from build123d import *

# Parameters (mm, degrees)
F0_W     = 28
F0_H     = 16
F1_DEPTH = 85
F2_W     = 23
F2_H     = 9
F2_H_2   = 7
F3_DEPTH = 25


with BuildPart() as f1:
    # F0 (on Front) → F1 (new body)
    with BuildSketch(Plane.XZ):
        Rectangle(F0_W, F0_H)
    extrude(amount=F1_DEPTH)

    # F2 (on face) → F3 (cut)
    with BuildSketch(Plane(origin=(0, 0, -8), x_dir=(1, 0, 0), z_dir=(0, 0, -1))):
        with Locations((0, 77.5)):
            Rectangle(F2_W, F2_H)
        with Locations((0, 65.5)):
            Rectangle(F2_W, F2_H)
        with Locations((0, 53.5)):
            Rectangle(F2_W, F2_H)
        with Locations((0, 41.5)):
            Rectangle(F2_W, F2_H)
        with Locations((0, 29.5)):
            Rectangle(F2_W, F2_H)
        with Locations((0, 17.5)):
            Rectangle(F2_W, F2_H)
        with Locations((0, 6.5)):
            Rectangle(F2_W, F2_H_2)
    extrude(amount=-F3_DEPTH, mode=Mode.SUBTRACT)


solid = f1.part
Can you work these out from the model? Positions are in its coordinate system, mm. A direction names the side the tool comes from. Round coordinates to 2 decimals unless told otherwise and drop trailing zeros. Loops run counter-clockwise (first coordinate to the right, second up) from the corner with the lowest first, then second, coordinate; pieces in that order, holes last. Notation, with made-up numbers: (69, -21.75) - (96, -21.75) arc R22 cw to (96, -6.75) - close; hole circle Ø8 at (41, 89). An arc over 180 degrees is marked (long way). Use CSV: the item, a comma, the result in double quotes. Start each with the question number.
1) For pin 1 Ø1.5 at (x, z) = (-5, -3) entering from +Y, with a flat end and sliding along its axis, tell me the tip position at first contact or that it passes through.
2) For faces 1 (the flat face through (0, -13, 0)), 2 (the flat face through (-13, -51, 8)), which set-ups out of +Z, -Z, +X, -X, +Y, -Y let a thin tool reach every point of the face, with its end or its side?
3) We'd pull the mould along X, two halves only. Please class faces 3 (the flat face through (-14, -42, 0)), 4 (the flat face through (0, 0, 0)), 5 (the flat face through (0, -25, 0)): released by +X, released by -X, zero draft, split by the parting line, or undercut.
4) Please list where this line runs through material, in increasing order: probe 1 along X at (y, z) = (-17, -4.75). Write a range as [from, to].
5) If we section it at B-B on x = 5: Count the separate pieces of the cut face and the enclosed holes in it, plus the area to 3 significant figures.
6) If we section it at A-A on y = -78: Write out the boundary of the cut face in (x, z).
Geometry results:
1,pin 1,"stops at y = 0"
2,face 1,"+Z, -Z"
2,face 2,"+Z, +X, -X, +Y, -Y"
3,face 3,"released by -X"
3,face 4,"zero draft"
3,face 5,"undercut"
4,probe 1,"x = [-14, -11.5], [11.5, 14]"
5,separate pieces,"8"
5,enclosed holes,"0"
5,area,"384 mm2"
6,outline,"(-14, -8) - (-11.5, -8) - (-11.5, 8) - (-14, 8) - close; (11.5, -8) - (14, -8) - (14, 8) - (11.5, 8) - close"
